Solid Edge part; units mm, degrees
sketch "Sketch1" plane through (0, 0, 0) normal (0, 0, 1) x (1, 0, 0)
  line L0 (-32.5, -3.5) -> (32.5, -3.5)
  line L1 (32.5, -3.5) -> (32.5, 3.5)
  line L2 (32.5, 3.5) -> (-32.5, 3.5)
  line L3 (-32.5, 3.5) -> (-32.5, -3.5)
extrude "Extrusionsausprägung_1" add sketch "Sketch1" along normal blind 2
hole "Bohrung_1" at (-26, 0, 2) direction (0, 0, -1) diameter 4.3 end up to next
hole "Hole1" at (26, 0, 2) direction (0, 0, -1) diameter 4.3 end up to next
hole "Bohrung_3" at (-5.5, 0, 2) direction (0, 0, -1) diameter 3.2 end up to next
hole "Hole2" at (5.5, 0, 2) direction (0, 0, -1) diameter 3.2 end up to next
properties material "Acryl, hoher Anschlag"
Verification items for the finished model (mm, model axes). Coordinates: 2 decimals unless noted, no trailing zeros. Loops run counter-clockwise (first coordinate to the right, second up) from the corner with the lowest first, then second, coordinate; pieces in that order, holes last. Notation, with made-up numbers: M 71,-4 L 122,-4 A13 cw 122,12 Z; hole C 66,39 d4. An arc over 180 degrees is marked long. One line per item, written item: value.
1. Section check D-D on x = -5.5. Record the cut outline in (y, z), plus the area to 3 significant figures.
Answers follow:
outline: M -3.5,0 L -1.6,0 L -1.6,2 L -3.5,2 Z; M 1.6,0 L 3.5,0 L 3.5,2 L 1.6,2 Z
area: 7.60 mm^2
2. Section check C-C on z = 1.3. Record the cut outline in (x, y), plus the area to 3 significant figures.
Answers follow:
outline: M -32.5,-3.5 L 32.5,-3.5 L 32.5,3.5 L -32.5,3.5 Z; hole C -26,0 d4.3; hole C -5.5,0 d3.2; hole C 5.5,0 d3.2; hole C 26,0 d4.3
area: 410 mm^2
3. Gauge pin test, flat end, axial feed: P1, Ø4, axis at x = -26, y = 0, coming from the +Z side. Record the tip position at first contact, or that the pin passes through.
Answers follow:
P1: through
4. Section check A-A on y = 0. Record the cut outline in (x, z).
Answers follow:
outline: M -32.5,0 L -28.15,0 L -28.15,2 L -32.5,2 Z; M -23.85,0 L -7.1,0 L -7.1,2 L -23.85,2 Z; M -3.9,0 L 3.9,0 L 3.9,2 L -3.9,2 Z; M 7.1,0 L 23.85,0 L 23.85,2 L 7.1,2 Z; M 28.15,0 L 32.5,0 L 32.5,2 L 28.15,2 Z
5. Mould release check, pull along Y, two halves, no side actions. Record for faces 1 (the flat face through (0, 3.5, 1)), 2 (the flat face through (0, 0, 0)), 3 (the cylindrical face through (-7.06, 0.35, 1.01)): pulls with the +Y half, pulls with the -Y half, needs draft (parallel to the pull), parting line crosses it, or undercut.
Answers follow:
face 1: pulls with the +Y half
face 2: needs draft
face 3: undercut
6. Section check B-B on x = -26. Record the cut outline in (y, z), plus the area to 3 significant figures.
Answers follow:
outline: M -3.5,0 L -2.15,0 L -2.15,2 L -3.5,2 Z; M 2.15,0 L 3.5,0 L 3.5,2 L 2.15,2 Z
area: 5.40 mm^2
7. Material ranges on line 1 along X through (y, z) = (0, 0.7); line 2 along Y through (x, z) = (26, 0.7); line 3 along Y through (x, z) = (5.5, 0.8), recorded low to high. Write a range as from..to.
Answers follow:
line 1: -32.5..-28.15, -23.85..-7.1, -3.9..3.9, 7.1..23.85, 28.15..32.5
line 2: -3.5..-2.15, 2.15..3.5
line 3: -3.5..-1.6, 1.6..3.5
